Could you check a few things on this model? Use its own coordinates, in mm. A direction names the side the tool comes from. Coordinates: 2 decimals unless noted, no trailing zeros. Loops run counter-clockwise (first coordinate to the right, second up) from the corner with the lowest first, then second, coordinate; pieces in that order, holes last. Notation, with made-up numbers: M 79,68.5 L 94,68.5 A33 ccw 94,101.5 Z; hole C 5,22.5 d4. An arc over 180 degrees is marked long. Use one line per item in the form item = value. Start each with the question number.
```python
from build123d import *

# Parameters (mm, degrees)
F0_W     = 50
F0_H     = 50
F1_DEPTH = 50
F2_W     = 33.4872
F2_H     = 34.45318
F3_DEPTH = 25
F4_W     = 18.03157
F4_H     = 16.849448
F5_DEPTH = 16.7


with BuildPart() as f1:
    # F0 (on Front) → F1 (new body)
    with BuildSketch(Plane.XZ):
        Rectangle(F0_W, F0_H)
    extrude(amount=F1_DEPTH)

    # F2 (on face) → F3 (join)
    with BuildSketch(Plane.XZ.offset(50)):
        Rectangle(F2_W, F2_H)
    extrude(amount=F3_DEPTH)

    # F4 (on face) → F5 (join, symmetric)
    with BuildSketch(Plane.XZ.offset(75)):
        Rectangle(F4_W, F4_H)
    extrude(amount=F5_DEPTH, both=True)


solid = f1.part
```
Item 1: For faces 1 (the flat face through (0, -62, -17.227)), 2 (the flat face through (-9.016, -83, 0)), 3 (the flat face through (-25, -25, 0)), 4 (the flat face through (0, -62, 17.227)), 5 (the flat face through (9.016, -83, 0)), which set-ups out of +Z, -Z, +X, -X, +Y, -Y let a thin tool reach every point of the face, with its end or its side?
Item 2: I want a section at B-B (z = 7). Write out the boundary of the cut face in (x, y).
Item 3: I want a section at C-C (y = -55.5). Write out the boundary of the cut face in (x, z), plus the area to 3 significant figures.
Item 4: Please list where these lines run through material, in increasing order: line 1 along Z through (x, y) = (-9, -72.5); line 2 along Y through (x, z) = (2.5, -10); line 3 along Z through (x, y) = (2.5, -87.5).
Item 5: I want a section at A-A (x = -2.5). Write out the boundary of the cut face in (y, z).
Item 6: I want a section at D-D (x = -13.5). Write out the boundary of the cut face in (y, z), plus the area to 3 significant figures.
Item 7: I'm going to push flat-ended pins straight in: P1, Ø5, axis at x = 4, y = -82.5, coming from the -Z side; P2, Ø4, axis at x = -4.5, z = 17.5, coming from the -Y side; P3, Ø1, axis at x = 13.5, y = -65, coming from the -Z side; P4, Ø1, axis at x = 10.5, z = -19.5, coming from the +Y side. Where does each tip first touch, or does it pass through?
Worked answers:
q1.face_1 = -Z, +X, -X, -Y
q1.face_2 = +Z, -Z, -X, -Y
q1.face_3 = +Z, -Z, -X, +Y, -Y
q1.face_4 = +Z, +X, -X, -Y
q1.face_5 = +Z, -Z, +X, -Y
q2.outline = M -25,-50 L -16.74,-50 L -16.74,-75 L -9.02,-75 L -9.02,-91.7 L 9.02,-91.7 L 9.02,-75 L 16.74,-75 L 16.74,-50 L 25,-50 L 25,0 L -25,0 Z
q3.outline = M -16.74,-17.23 L 16.74,-17.23 L 16.74,17.23 L -16.74,17.23 Z
q3.area = 1,150 mm²
q4.line_1 = -17.23 to 17.23
q4.line_2 = -75 to 0
q4.line_3 = -8.42 to 8.42
q5.outline = M -91.7,-8.42 L -75,-8.42 L -75,-17.23 L -50,-17.23 L -50,-25 L 0,-25 L 0,25 L -50,25 L -50,17.23 L -75,17.23 L -75,8.42 L -91.7,8.42 Z
q6.outline = M -75,-17.23 L -50,-17.23 L -50,-25 L 0,-25 L 0,25 L -50,25 L -50,17.23 L -75,17.23 Z
q6.area = 3,360 mm²
q7.P1 = -8.42
q7.P2 = -75
q7.P3 = -17.23
q7.P4 = 0
